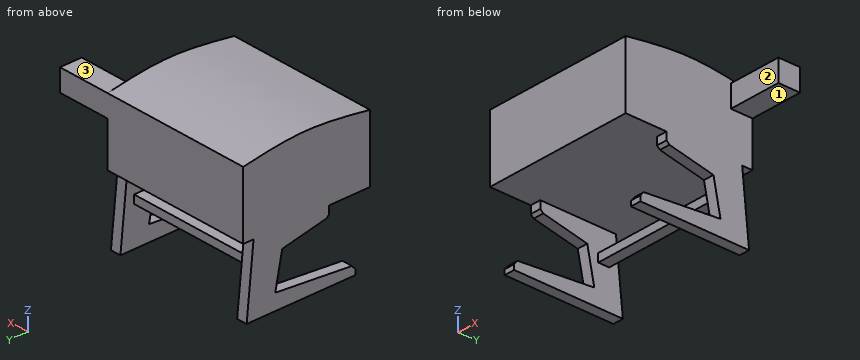
from build123d import *

# Parameters (mm, degrees)
F1_DEPTH = 1000
F2_W     = 145
F2_H     = 145
F3_DEPTH = 350
F5_DEPTH = 70
F8_W     = 73.3011215925
F8_H     = 54.268091917
F9_DEPTH = 860


with BuildPart() as f1:
    # F0 (on Right) → F1 (new body)
    with BuildSketch(Plane.YZ):
        with BuildLine():
            Line((-535.786010325, -296.8136846698), (314.213989675, -296.8136846698))
            Line((314.213989675, -296.8136846698), (314.213989675, 143.1863153302))
            add(Edge.make_bspline(
                [(314.213989675, 143.1863153302), (176.5867674254, 165.9648621816), (-101.8189451009, 210.2443102405), (-390.0428643628, 166.3108724655), (-535.786010325, 143.1863153302)],
                knots=[0, 0, 0, 0, 0.4943481252, 1, 1, 1, 1], degree=3))
            Line((-535.786010325, 143.1863153302), (-535.786010325, -296.8136846698))
        make_face()
    extrude(amount=F1_DEPTH)

    # F2 (on face) → F3 (join)
    with BuildSketch(Plane.YZ.offset(1000)):
        with Locations((241.713989675, 70.6863153302)):
            Rectangle(F2_W, F2_H)
    extrude(amount=F3_DEPTH)

    # F7: F5 across plane


with BuildPart() as f5:
    # F4 (on face) → F5 (new body)
    with BuildSketch(Plane.YZ.offset(1000)):
        Polygon((291.2076711655, -761.8098408201), (244.7297275066, -296.8136846698), (-262.2444331646, -296.8136846698), (-262.2444331646, -346.7207700231), (-242.4782663584, -364.9664670446), (52.4934381247, -424.2648929575), (99.6281057596, -656.8972617605), (-414.2917096615, -700.9909302213), (-437.098801136, -728.3594757536), (-437.098801136, -761.8098408201), align=None)
    extrude(amount=-F5_DEPTH)


with BuildPart() as f1_1:
    add(f1.part)
    add(f5.part.mirror(Plane(origin=(500, -120.4719590478, -66.200953195), x_dir=(0, 1, 0), z_dir=(-1, 0, 0))))


    add(f5.part)  # F9 merges F5
    # F8 (on face) → F9 (join, through all)
    with BuildSketch(Plane(origin=(930, 0, 0), x_dir=(0, -1, 0), z_dir=(-1, 0, 0))):
        with Locations((-162.7628132701, -476.7469912767)):
            Rectangle(F8_W, F8_H)
    extrude(amount=F9_DEPTH)


solid = f1_1.part
Design review of the part built by this model. Coordinates are the model's own, in mm. Face numbers are marked on the shaded views. A direction names the side the tool comes from. Round coordinates to 2 decimals unless told otherwise and drop trailing zeros. Write each loop counter-clockwise with the first axis right and the second up, starting at its lowest first coordinate (ties: lowest second). Pieces come first, ordered by that corner, then holes. Notation, with made-up numbers: (39.5, -15.5) - (85.5, -15.5) arc R21 cw to (85.5, 2.5) - close; hole circle Ø4 at (15, 15). An arc over 180 degrees is marked (long way). Use a Markdown table: item, result. Add a question column.
1. Wall thickness on probe 1 along X at (y, z) = (-189, -336.5); probe 2 along X at (y, z) = (-224.5, 32); probe 3 along Y at (x, z) = (716.5, -482): over which ranges is each line inside the solid? List them lowest first.
2. We need section A-A (z = -573). State the section outline as (x, y) points, then the cut area to 3 significant figures.
3. Clearance check with flat-ended pins moving along their axes: pin 1 (1 mm diameter, centred on x = 800.5, y = 147, fed in from +Z); pin 2 (12 mm diameter, centred on x = 148.5, y = 191, fed in from +Z); pin 3 (22 mm diameter, centred on x = 352, y = 157.5, fed in from -Z); pin 4 (1 mm diameter, centred on y = -339.5, z = -16.5, fed in from -X). State where each tip first meets the part, or that it passes through.
4. We need section B-B (x = 1190). State the section outline as (y, z) points.
5. We need section D-D (z = 126). State the section outline as (x, y) points, then the cut area to 3 significant figures.
6. We need section C-C (y = -165). Count the separate pieces of the cut face and the enclosed holes in it, then the cut area to 3 significant figures.
7. For the marked faces 1, 2 and 3, list the 3-axis set-ups (+Z, -Z, +X, -X, +Y, -Y) from which the entire face can be reached by the end or side of a thin tool; tool diameter is ignored.
Output:
| question | item | result |
|---|---|---|
| 1 | probe 1 | x = 0 to 70, 930 to 1000 |
| 1 | probe 2 | x = 0 to 1000 |
| 1 | probe 3 | y = 126.11 to 199.41 |
| 2 | outline | (0, 82.63) - (70, 82.63) - (70, 272.34) - (0, 272.34) - close; (930, 82.63) - (1000, 82.63) - (1000, 272.34) - (930, 272.34) - close |
| 2 | area | 26,600 mm2 |
| 3 | pin 1 | stops at z = 169.1 |
| 3 | pin 2 | stops at z = 163.67 |
| 3 | pin 3 | stops at z = -503.88 |
| 3 | pin 4 | stops at x = 0 |
| 4 | outline | (169.21, -1.81) - (314.21, -1.81) - (314.21, 143.19) - (169.21, 143.19) - close |
| 5 | outline | (0, -535.79) - (1000, -535.79) - (1000, 169.21) - (1350, 169.21) - (1350, 314.21) - (0, 314.21) - close |
| 5 | area | 901,000 mm2 |
| 6 | separate pieces | 3 |
| 6 | enclosed holes | 0 |
| 6 | area | 507,000 mm2 |
| 7 | face 1 | -Z, +X, +Y, -Y |
| 7 | face 2 | +Z, -Z, +X, -Y |
| 7 | face 3 | +Z, +X, +Y, -Y |
